Input: part model. Units: mm. Frame: model coordinates. Face numbers are marked on the shaded views. Round coordinates to 2 decimals unless told otherwise and drop trailing zeros. Loops run counter-clockwise (first coordinate to the right, second up) from the corner with the lowest first, then second, coordinate; pieces in that order, holes last. Notation, with made-up numbers: (42.25, 33) - (67.25, 33) arc R18 cw to (67.25, 59) - close; hole circle Ø5 at (-29, 25). An arc over 180 degrees is marked (long way). One line per question, with ' | ' between items. Start each with the question number.
Item 1: Section B-B, the plane y = -23. Return loops of the section in (x, z), plus the area to 3 significant figures.
Item 2: Material intervals for line 1 along Z through (x, y) = (-10.5, -19.5); line 2 along X through (y, z) = (-7.25, -59); line 3 along Y through (x, z) = (117, -61), sorted ascending.
Item 3: Section A-A, the plane z = 92.5. Return loops of the section in (x, y), plus the area to 3 significant figures.
Item 4: Draft query along X for the marked faces 1, 2 and 3. Return one class per face: pulls with the +X half, pulls with the -X half, needs draft (parallel to the pull), parting line crosses it, or undercut.
Item 5: Section C-C, the plane x = 12.5. Return loops of the section in (y, z), plus the area to 3 significant figures.
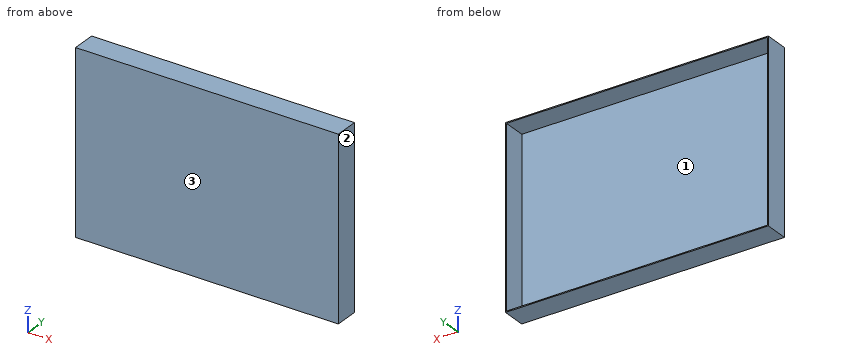
```python
from build123d import *

# Parameters (mm, degrees)
F0_W     = 315
F0_H     = 215
F0_W_2   = 312.6
F0_H_2   = 212.6
F1_DEPTH = 28.5
F2_W     = 312.6
F2_H     = 212.6
F3_DEPTH = 1.5


with BuildPart() as f1:
    # F0 (on Front) → F1 (new body)
    with BuildSketch(Plane.XZ):
        with Locations((-7.5, -1.3)):
            Rectangle(F0_W, F0_H)
        with Locations((-7.5, -1.3)):
            Rectangle(F0_W_2, F0_H_2, mode=Mode.SUBTRACT)
    extrude(amount=F1_DEPTH)

    # F2 (on face) → F3 (join)
    with BuildSketch(Plane.XZ.offset(28.5)):
        with Locations((-7.5, -1.3)):
            Rectangle(F2_W, F2_H)
    extrude(amount=-F3_DEPTH)


solid = f1.part
```
Return value:
1) outline: (-165, -108.8) - (150, -108.8) - (150, 106.2) - (-165, 106.2) - close; hole (-163.8, -107.6) - (148.8, -107.6) - (148.8, 105) - (-163.8, 105) - close | area: 1,270 mm2
2) line 1: -108.8 to -107.6, 105 to 106.2 | line 2: -165 to -163.8, 148.8 to 150 | line 3: -28.5 to -27
3) outline: (-165, -28.5) - (150, -28.5) - (150, 0) - (148.8, 0) - (148.8, -27) - (-163.8, -27) - (-163.8, 0) - (-165, 0) - close | area: 537 mm2
4) face 1: undercut | face 2: pulls with the +X half | face 3: needs draft
5) outline: (-28.5, -108.8) - (0, -108.8) - (0, -107.6) - (-27, -107.6) - (-27, 105) - (0, 105) - (0, 106.2) - (-28.5, 106.2) - close | area: 387 mm2
